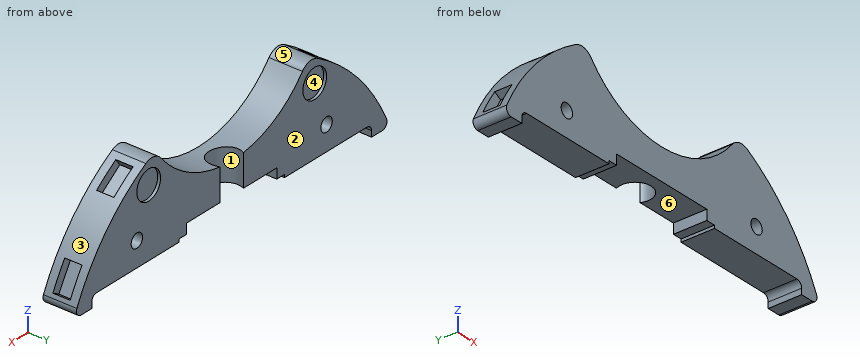
```python
from build123d import *

# Parameters (mm, degrees)
BOSS_EXTRUDE1_DEPTH  = 5.8
SOLENOID_PLACEMENT_W = 38
SOLENOID_PLACEMENT_H = 64
CUT_EXTRUDE1_DEPTH   = 103.481998419
SKETCH6_R            = 2.4
CUT_EXTRUDE6_DEPTH   = 103.481998419
CUT_EXTRUDE3_DEPTH   = 103.481998419
FILLET1_R            = 2
CUT_EXTRUDE7_DEPTH   = 3
SKETCH11_R           = 5.5
CUT_EXTRUDE8_DEPTH   = 72.028583754
SKETCH12_W           = 44.5
SKETCH12_H           = 65
CUT_EXTRUDE9_DEPTH   = 92.53668667
SKETCH13_R           = 5
CUT_EXTRUDE10_DEPTH  = 1


with BuildPart() as part:
    # Sketch1 → Boss-Extrude1 (new, symmetric)
    with BuildSketch(Plane(origin=(0, 0, 0), x_dir=(1, 0, 0), z_dir=(0, 1, 0))):
        with BuildLine():
            ThreePointArc((36.224522061, -62.223661106), (0, 72), (-36.224522061, -62.223661106))
            ThreePointArc((-36.224522061, -62.223661106), (-32.797800029, -62.818856853), (-29.811944095, -61.035223988))
            ThreePointArc((-29.811944095, -61.035223988), (0, -46.75), (29.811944095, -61.035223988))
            ThreePointArc((29.811944095, -61.035223988), (32.797800029, -62.818856853), (36.224522061, -62.223661106))
        make_face()
    extrude(amount=BOSS_EXTRUDE1_DEPTH, both=True)

    # solenoid placement → Cut-Extrude1 (cut, through all)
    with BuildSketch(Plane(origin=(0, 5.8, 0), x_dir=(1, 0, 0), z_dir=(0, 1, 0))):
        with Locations((0, -4)):
            Rectangle(SOLENOID_PLACEMENT_W, SOLENOID_PLACEMENT_H)
    extrude(amount=-CUT_EXTRUDE1_DEPTH, mode=Mode.SUBTRACT)

    # Sketch6 → Cut-Extrude6 (cut, through all)
    with BuildSketch(Plane(origin=(0, 5.8, 0), x_dir=(1, 0, 0), z_dir=(0, 1, 0))):
        with Locations(Location((40, -40, 0), (0, 0, 90))):
            Circle(SKETCH6_R)
        with Locations(Location((-40, -40, 0), (0, 0, 270))):
            Circle(SKETCH6_R)
    extrude(amount=-CUT_EXTRUDE6_DEPTH, mode=Mode.SUBTRACT)

    # Sketch3 → Cut-Extrude3 (cut, through all)
    with BuildSketch(Plane(origin=(0, 5.8, 0), x_dir=(1, 0, 0), z_dir=(0, 1, 0))):
        Polygon((-72, -27.5), (-59, -27.5), (-59, -31.5), (59, -31.5), (59, -27.5), (72, -27.5), (72, 31.5), (72, 72), (-72, 72), (-72, 31.5), align=None)
    extrude(amount=-CUT_EXTRUDE3_DEPTH, mode=Mode.SUBTRACT)

    # Fillet1
    fillet1_edges = [part.edges().sort_by_distance(p)[0] for p in [
        (66.541340534, 0, 27.5),
        (-66.541340534, 0, 27.5),
        (59, 0, 31.5),
        (-59, 0, 31.5),
    ]]
    fillet(fillet1_edges, radius=FILLET1_R)

    # Sketch9 → Cut-Extrude7 (cut, symmetric)
    with BuildSketch(Plane(origin=(0, 0, 0), x_dir=(1, 0, 0), z_dir=(0, 1, 0))):
        with BuildLine():
            Line((-64.703295733, -31.582962517), (-62.191822062, -30.132962517))
            Line((-62.191822062, -30.132962517), (-57.191822062, -38.793216555))
            Line((-57.191822062, -38.793216555), (-59.703295733, -40.243216555))
            ThreePointArc((-59.703295733, -40.243216555), (-62.353829072, -36), (-64.703295733, -31.582962517))
        make_face()
        with BuildLine():
            Line((-46.263453759, -55.169673248), (-44.558876527, -52.823523965))
            Line((-44.558876527, -52.823523965), (-36.468706583, -58.701376488))
            Line((-36.468706583, -58.701376488), (-38.173283815, -61.047525771))
            ThreePointArc((-38.173283815, -61.047525771), (-42.320538165, -58.249223595), (-46.263453759, -55.169673248))
        make_face()
        with BuildLine():
            Line((38.173283815, -61.047525771), (36.468706583, -58.701376488))
            Line((36.468706583, -58.701376488), (44.558876527, -52.823523965))
            Line((44.558876527, -52.823523965), (46.263453759, -55.169673248))
            ThreePointArc((46.263453759, -55.169673248), (42.320538165, -58.249223595), (38.173283815, -61.047525771))
        make_face()
        with BuildLine():
            Line((59.703295733, -40.243216555), (57.191822062, -38.793216555))
            Line((57.191822062, -38.793216555), (62.191822062, -30.132962517))
            Line((62.191822062, -30.132962517), (64.703295733, -31.582962517))
            ThreePointArc((64.703295733, -31.582962517), (62.353829072, -36), (59.703295733, -40.243216555))
        make_face()
    extrude(amount=CUT_EXTRUDE7_DEPTH, both=True, mode=Mode.SUBTRACT)

    # Sketch11 → Cut-Extrude8 (cut, through all)
    with BuildSketch(Plane(origin=(0, 0, 36), x_dir=(-1, 0, 0), z_dir=(0, 0, -1))):
        with Locations((0, 3.4)):
            Circle(SKETCH11_R)
    extrude(amount=-CUT_EXTRUDE8_DEPTH, mode=Mode.SUBTRACT)

    # Sketch12 → Cut-Extrude9 (cut, through all)
    with BuildSketch(Plane(origin=(0, 5.8, 0), x_dir=(1, 0, 0), z_dir=(0, 1, 0))):
        Rectangle(SKETCH12_W, SKETCH12_H)
    extrude(amount=-CUT_EXTRUDE9_DEPTH, mode=Mode.SUBTRACT)

    # Sketch13 → Cut-Extrude10 (cut)
    with BuildSketch(Plane(origin=(0, 5.8, 0), x_dir=(1, 0, 0), z_dir=(0, 1, 0))):
        with Locations(Location((-35, -55, 0), (0, 0, 270))):
            Circle(SKETCH13_R)
        with Locations(Location((35, -55, 0), (0, 0, 90))):
            Circle(SKETCH13_R)
    extrude(amount=-CUT_EXTRUDE10_DEPTH, mode=Mode.SUBTRACT)


solid = part.part
```
Read the model definition and answer for the solid it produces. Units are mm, in the model's axes. Face numbers are marked on the shaded views. A direction names the side the tool comes from. Coordinates: 2 decimals unless noted, no trailing zeros. Loops run counter-clockwise (first coordinate to the right, second up) from the corner with the lowest first, then second, coordinate; pieces in that order, holes last. Notation, with made-up numbers: (17, -24.5) - (29, -24.5) arc R22 ccw to (29, 1.5) - close; hole circle Ø11 at (74.5, -6.75). An arc over 180 degrees is marked (long way). Answer in a Markdown table with one row per item.
1. Determine the mould class of the marked faces 1, 2 and 3 for opening direction X: +X half, -X half, draft (parallel to the pull), parting line (faces both ways), or undercut.
Conclusion:
| item | result |
|---|---|
| face 1 | undercut |
| face 2 | draft |
| face 3 | +X half |
2. Given pin 1 (3 mm diameter, centred on x = 20.5, y = -2.5, fed in from +Z); pin 2 (2.5 mm diameter, centred on x = -21.5, y = 3, fed in from -Z); pin 3 (1 mm diameter, centred on y = -1, z = 48, fed in from +X); pin 4 (6 mm diameter, centred on x = -4.5, z = 53, fed in from +Y), each flat-ended and moving along its own axis, determine where each tip first touches the part or whether it passes through.
Conclusion:
| item | result |
|---|---|
| pin 1 | stops at z = 53.71 |
| pin 2 | stops at z = 31.5 |
| pin 3 | stops at x = 54.11 |
| pin 4 | passes through |
3. Find section A-A, the plane x = 35. Write down the section's boundary in (y, z).
Conclusion:
| item | result |
|---|---|
| outline | (-5.8, 31.5) - (5.8, 31.5) - (5.8, 50) - (4.8, 50) - (4.8, 60) - (5.8, 60) - (5.8, 62.73) - (-5.8, 62.73) - close |
4. Find section C-C, the plane x = -17. Write down the section's boundary in (y, z), then the cut area to 3 significant figures.
Conclusion:
| item | result |
|---|---|
| outline | (-5.8, 36) - (5.8, 36) - (5.8, 50.74) - (-5.8, 50.74) - close |
| area | 171 mm² |
5. Which of the six approach directions +Z, -Z, +X, -X, +Y, -Y give full straight-line access (tool end or side, diameter ignored) to the marked faces 4, 5 and 6?
Conclusion:
| item | result |
|---|---|
| face 4 | +Y |
| face 5 | +Z, +Y, -Y |
| face 6 | -Z, +Y, -Y |
6. Find section B-B, the plane x = -1. Write down the section's boundary in (y, z).
Conclusion:
| item | result |
|---|---|
| outline | (-5.8, 36) - (-2.01, 36) - (-2.01, 46.76) - (-5.8, 46.76) - close |
7. Straight lines are drawn through the part: line 1 (X direction, y = 3.4, z = 38.5); line 2 (X direction, y = 5, z = 55); line 3 (Y direction, x = 39, z = 54.5). For each, find the intervals that lie inside material, in ascending order.
Conclusion:
| item | result |
|---|---|
| line 1 | x = -60.84 to -41.87, -38.13 to -5.5, 5.5 to 38.13, 41.87 to 60.84 |
| line 2 | x = -46.47 to -40, -30 to -23.73, 23.73 to 30, 40 to 46.47 |
| line 3 | y = -5.8 to 4.8 |
